Autodesk Inventor part; units mm, degrees
ref_plane "YZ Plane" through (0, 0, 0) normal (1, 0, 0) x (0, 1, 0)
ref_plane "XZ Plane" through (0, 0, 0) normal (0, 1, 0) x (-1, 0, 0)
ref_plane "XY Plane" through (0, 0, 0) normal (0, 0, 1) x (1, 0, 0)
sketch "Sketch1" plane through (0, 0, 0) normal (0, 0, 1) x (1, 0, 0)
  circle A0 centre (0, 0) radius 11
  dimension "d0" = 22
extrude "Extrusion1" add sketch "Sketch1" along normal blind 0.9
sketch "Sketch2" plane through (0, 0, 0.9) normal (0, 0, 1) x (1, 0, 0)
  circle A0 centre (0, 0) radius 11
  point P0 (9.64, 0)
  dimension "d3" = 9.64
hole "Hole1" at (9.64, 0, 0.9) direction (0, 0, -1) diameter 1.181 depth 8
pattern_circular "Circular Pattern1" count 3 over 360 about axis through (0, 0, -10) along (0, 0, 1) of "Hole1"
properties part number "PCB"
Could you check a few things on this model? Use its own coordinates, in mm. Round coordinates to 2 decimals unless told otherwise and drop trailing zeros. Write each loop counter-clockwise with the first axis right and the second up, starting at its lowest first coordinate (ties: lowest second). Pieces come first, ordered by that corner, then holes. Notation, with made-up numbers: (21, 48) - (40, 48) arc R16 cw to (40, 57) - close; hole circle Ø4 at (80.5, 30). An arc over 180 degrees is marked (long way). Put each result on its own line as item: value. Start each with the question number.
(1) I want a section at D-D, the plane y = -4. Please give me the cut outline in (x, z).
(2) I want a section at B-B, the plane x = 9.64. Please give me the cut outline in (y, z), plus the area to 3 significant figures.
(3) I want a section at C-C, the plane x = -4.82. Please give me the cut outline in (y, z).
(4) I need wall thicknesses on probe 1 along X at (y, z) = (-8, 0.65); probe 2 along Y at (x, z) = (-5, 0.8); probe 3 along Y at (x, z) = (9.64, 0.2). Which ranges of each line are inside material? Lowest first, please.
(5) I want a section at A-A, the plane y = 0. Please give me the cut outline in (x, z), plus the area to 3 significant figures.
(6) Thinking about a two-plate mould opening in Y: for faces 1 (the cylindrical face through (10.216, 0.128, 0.444)), 2 (the cylindrical face through (-2.38, 10.74, 0.44)), 3 (the flat face through (0, 0, 0.9)), which applies, released by +Y, released by -Y, zero draft, split by the parting line, or undercut?
Here are the results:
1. outline: (-10.25, 0) - (10.25, 0) - (10.25, 0.9) - (-10.25, 0.9) - close
2. outline: (-5.3, 0) - (-0.59, 0) - (-0.59, 0.9) - (-5.3, 0.9) - close; (0.59, 0) - (5.3, 0) - (5.3, 0.9) - (0.59, 0.9) - close
2. area: 8.47 mm^2
3. outline: (-9.89, 0) - (-8.94, 0) - (-8.94, 0.9) - (-9.89, 0.9) - close; (-7.76, 0) - (7.76, 0) - (7.76, 0.9) - (-7.76, 0.9) - close; (8.94, 0) - (9.89, 0) - (9.89, 0.9) - (8.94, 0.9) - close
4. probe 1: x = -7.55 to -5.3, -4.34 to 7.55
4. probe 2: y = -9.8 to -8.91, -7.79 to 7.79, 8.91 to 9.8
4. probe 3: y = -5.3 to -0.59, 0.59 to 5.3
5. outline: (-11, 0) - (9.05, 0) - (9.05, 0.9) - (-11, 0.9) - close; (10.23, 0) - (11, 0) - (11, 0.9) - (10.23, 0.9) - close
5. area: 18.7 mm^2
6. face 1: undercut
6. face 2: split by the parting line
6. face 3: zero draft
